For this review, take the finished solid that the model builds, in its own axes (mm). A direction names the side the tool comes from. Round coordinates to 2 decimals unless told otherwise and drop trailing zeros. Loops run counter-clockwise (first coordinate to the right, second up) from the corner with the lowest first, then second, coordinate; pieces in that order, holes last. Notation, with made-up numbers: (-23.5, -5.75) -> (20.5, -5.75) arc R16 ccw to (20.5, 8.25) -> close; hole circle Ø3 at (85, 41). An arc over 180 degrees is marked (long way). Write each question's results on one line, items separated by ' | '.
```python
from build123d import *

# Parameters (mm, degrees)
SKETCH_1_R               = 10
SKETCH_1_R_2             = 3
EXTRUDE_1_DEPTH          = 12
CUT_EXTRUDE_START        = 6
SKETCH_2_R               = 5.05
CUT_EXTRUDE_1_DEPTH      = 12
PATTERN_CIRCULAR_1_COUNT = 4


with BuildPart() as part:
    # 草图1 → 凸台-拉伸1 (new body)
    with BuildSketch(Plane(origin=(0, 0, 0), x_dir=(1, 0, 0), z_dir=(0, 1, 0))):
        with Locations(Location((0, 0, 0), (0, 0, 270))):
            Circle(SKETCH_1_R)
        with Locations(Location((0, 0, 0), (0, 0, 270))):
            Circle(SKETCH_1_R_2, mode=Mode.SUBTRACT)
    extrude(amount=EXTRUDE_1_DEPTH)

    # 草图2 → 切除-拉伸1 (cut)
    with BuildSketch(Plane.XY.offset(CUT_EXTRUDE_START)):
        with Locations(Location((0, 6, 0), (0, 0, 180))):
            Circle(SKETCH_2_R)
    cut_extrude_1 = extrude(amount=CUT_EXTRUDE_1_DEPTH, mode=Mode.SUBTRACT)

    # 阵列(圆周)1: 切除-拉伸1 ×4 about axis
    pattern_circular_1_axis = Axis((0, 0, 0), (0, 1, 0))
    for i in range(1, PATTERN_CIRCULAR_1_COUNT):
        add(cut_extrude_1.rotate(pattern_circular_1_axis, i * 360 / PATTERN_CIRCULAR_1_COUNT), mode=Mode.SUBTRACT)


solid = part.part
```
1. To check wall thickness, follow probe 1 along Y at (x, z) = (8.4, 0); probe 2 along X at (y, z) = (4, 4); probe 3 along X at (y, z) = (4, -6.75). State the ranges of each line that lie inside material, in increasing order.
Values found:
probe 1: y = 0 to 0.95, 11.05 to 12 | probe 2: x = -6 to 6 | probe 3: x = -7.38 to -4.64, 4.64 to 7.38
2. Consider section B-B (z = 0). State the section outline as (x, y) points, plus the area to 3 significant figures.
Values found:
outline: (-10, 0) -> (-3, 0) -> (-3, 12) -> (-10, 12) -> (-10, 11.05) -> (-6, 11.05) -> (-6, 0.95) -> (-10, 0.95) -> close; (3, 0) -> (10, 0) -> (10, 0.95) -> (6, 0.95) -> (6, 11.05) -> (10, 11.05) -> (10, 12) -> (3, 12) -> close | area: 87.2 mm2
3. Consider section D-D (z = 7.5). State the section outline as (x, y) points.
Values found:
outline: (-6.61, 0) -> (6.61, 0) -> (6.61, 12) -> (-6.61, 12) -> close; hole circle Ø10.1 at (0, 6)
4. For pin 1 (5.5 mm diameter, centred on x = 0, z = 0, fed in from -Y); pin 2 (2 mm diameter, centred on x = 8, y = 10, fed in from -Z); pin 3 (3 mm diameter, centred on x = -3, y = 3, fed in from +Z); pin 4 (4 mm diameter, centred on x = -3, y = 6, fed in from -Z), all flat-tipped, find the tip position at first contact; note any pin that passes through.
Values found:
pin 1: passes through | pin 2: stops at z = -7.14 | pin 3: stops at z = 9.69 | pin 4: stops at z = -6
5. Tool access review of faces 1 (the face through (-7.528, 5.778, 5.045)), 2 (the face through (5.045, 5.778, 7.528)), 3 (the face through (7.528, 5.778, -5.045)), 4 (the face through (0, 6, -6)): name each direction out of +Z, -Z, +X, -X, +Y, -Y from which nothing blocks a thin tool from reaching the whole face with its end or side.
Values found:
face 1: -X | face 2: +Z | face 3: +X | face 4: -Z
6. Consider section C-C (y = 8.5). State the section outline as (x, z) points, plus the area to 3 significant figures.
Values found:
outline: (-8.99, -4.39) arc R10 ccw to (-4.39, -8.99) -> (-4.39, -6) -> (4.39, -6) -> (4.39, -8.99) arc R10 ccw to (8.99, -4.39) -> (6, -4.39) -> (6, 4.39) -> (8.99, 4.39) arc R10 ccw to (4.39, 8.99) -> (4.39, 6) -> (-4.39, 6) -> (-4.39, 8.99) arc R10 ccw to (-8.99, 4.39) -> (-6, 4.39) -> (-6, -4.39) -> close; hole circle Ø6 at (0, 0) | area: 157 mm2
7. Draft analysis for pull direction X (two halves, no side actions). For faces 5 (the face through (-5.045, 5.778, -7.528)), 6 (the face through (2.4, 12, 2.1)), 7 (the face through (0, 6, 6)), 8 (the face through (-6, 6, 0)), state which applies: released by +X, released by -X, zero draft, split by the parting line, or undercut.
Values found:
face 5: undercut | face 6: zero draft | face 7: undercut | face 8: released by -X
8. Consider section A-A (x = 0). State the section outline as (y, z) points, plus the area to 3 significant figures.
Values found:
outline: (0, -10) -> (0.95, -10) -> (0.95, -6) -> (11.05, -6) -> (11.05, -10) -> (12, -10) -> (12, -3) -> (0, -3) -> close; (0, 3) -> (12, 3) -> (12, 10) -> (11.05, 10) -> (11.05, 6) -> (0.95, 6) -> (0.95, 10) -> (0, 10) -> close | area: 87.2 mm2
